Check sheet for the drawn part. Datum: minimum x, y, z corner. Units: mm. Give positions to 0.01 mm unless a question says otherwise; leave off trailing zeros. Loops run counter-clockwise (first coordinate to the right, second up) from the corner with the lowest first, then second, coordinate; pieces in that order, holes last. Notation, with made-up numbers: (14, 85) -> (58, 85) arc R25 cw to (58, 117) -> close; hole circle Ø3 at (30.5, 57.25). An arc over 180 degrees is marked (long way). One line per question, with ' | ' between items.
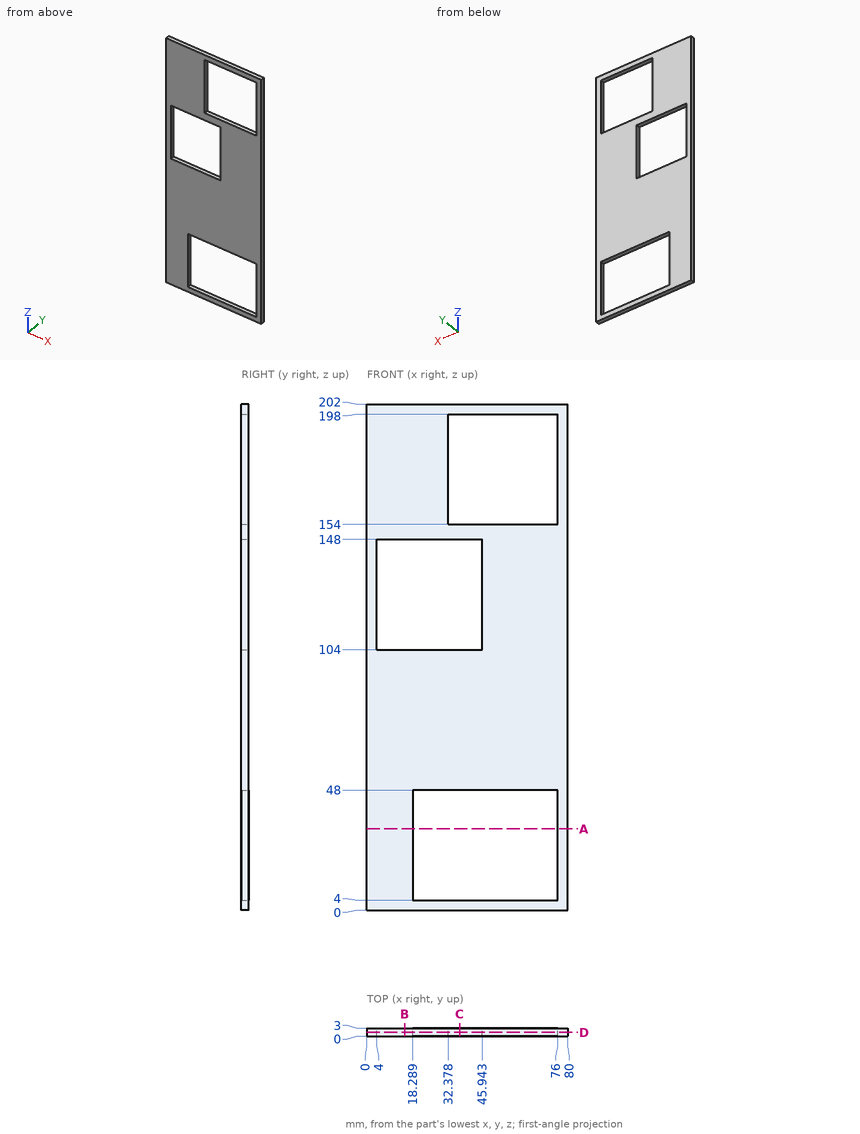
Item 1: Sectioned sample at D-D (y = 1.4). Record the cut outline in (x, z).
Result:
outline: (0, 0) -> (80, 0) -> (80, 202) -> (0, 202) -> close; hole (4, 104) -> (45.94, 104) -> (45.94, 148) -> (4, 148) -> close; hole (18.29, 4) -> (76, 4) -> (76, 48) -> (18.29, 48) -> close; hole (32.38, 154) -> (76, 154) -> (76, 198) -> (32.38, 198) -> close
Item 2: Sectioned sample at C-C (x = 37). Record the cut outline in (y, z), plus the area to 3 significant figures.
Result:
outline: (0, 0) -> (3, 0) -> (3, 4) -> (0, 4) -> close; (0, 48) -> (3, 48) -> (3, 104) -> (0, 104) -> close; (0, 148) -> (3, 148) -> (3, 154) -> (0, 154) -> close; (0, 198) -> (3, 198) -> (3, 202) -> (0, 202) -> close | area: 210 mm2
Item 3: Scan lines: probe 1 along Z at (x, y) = (61.5, 2.4); probe 2 along Z at (x, y) = (40, 2.1); probe 3 along Z at (x, y) = (20, 0.9). Record each from-to range of solid material in increasing order.
Result:
probe 1: 0 to 4, 48 to 154, 198 to 202 | probe 2: 0 to 4, 48 to 104, 148 to 154, 198 to 202 | probe 3: 0 to 4, 48 to 104, 148 to 202
Item 4: Sectioned sample at A-A (z = 32.5). Record the cut outline in (x, y).
Result:
outline: (0, 0) -> (18.29, 0) -> (18.29, 3) -> (0, 3) -> close; (76, 0) -> (80, 0) -> (80, 3) -> (76, 3) -> close
Item 5: Sectioned sample at B-B (x = 15). Record the cut outline in (y, z), plus the area to 3 significant figures.
Result:
outline: (0, 0) -> (3, 0) -> (3, 104) -> (0, 104) -> close; (0, 148) -> (3, 148) -> (3, 202) -> (0, 202) -> close | area: 474 mm2
